```python
from build123d import *

# Parameters (mm, degrees)
EXTRUDE_1_DEPTH          = 40
SKETCH_2_R               = 3
CUT_EXTRUDE_1_DEPTH      = 14
SKETCH_3_R               = 4.25
CUT_EXTRUDE_2_DEPTH      = 33
CUT_EXTRUDE_2_DEPTH_BACK = 33
FILLET_1_R               = 15


with BuildPart() as part:
    # 草圖1 → 填料-伸長1 (new body)
    with BuildSketch(Plane.XY):
        with BuildLine():
            Line((-23, 35), (-32, 0))
            Line((-32, 0), (-25, 0))
            ThreePointArc((-25, 0), (0, 25), (25, 0))
            Line((25, 0), (32, 0))
            Line((32, 0), (23, 35))
            Line((23, 35), (23, 39))
            Line((23, 39), (-23, 39))
            Line((-23, 39), (-23, 35))
        make_face()
    extrude(amount=EXTRUDE_1_DEPTH)

    # 草圖2 → 除料-伸長1 (cut)
    with BuildSketch(Plane(origin=(0, 39, 0), x_dir=(1, 0, 0), z_dir=(0, 1, 0))):
        with Locations((-12, -20)):
            Circle(SKETCH_2_R)
        with Locations((12, -20)):
            Circle(SKETCH_2_R)
    extrude(amount=-CUT_EXTRUDE_1_DEPTH, mode=Mode.SUBTRACT)

    # 草圖3 → 除料-伸長2 (cut, two sides)
    with BuildSketch(Plane(origin=(0, 0, 0), x_dir=(0, 0, -1), z_dir=(1, 0, 0))) as cut_extrude_2_sk:
        with Locations((-20, 12)):
            Circle(SKETCH_3_R)
    extrude(amount=CUT_EXTRUDE_2_DEPTH, mode=Mode.SUBTRACT)
    extrude(cut_extrude_2_sk.sketch, amount=-CUT_EXTRUDE_2_DEPTH_BACK, mode=Mode.SUBTRACT)

    # 圓角1
    fillet_1_edges = [part.edges().sort_by_distance(p)[0] for p in [
        (-28.5, 0, 0),
        (-28.5, 0, 40),
        (28.5, 0, 40),
        (28.5, 0, 0),
    ]]
    fillet(fillet_1_edges, radius=FILLET_1_R)


solid = part.part
```
CAD build for the part. Positions are in the model's coordinates, mm. A direction names the side the tool comes from. Round coordinates to 2 decimals unless told otherwise and drop trailing zeros. Write each loop counter-clockwise with the first axis right and the second up, starting at its lowest first coordinate (ties: lowest second). Pieces come first, ordered by that corner, then holes. Notation, with made-up numbers: (-13, 5) -> (1, 5) arc R6 ccw to (1, 11) -> close; hole circle Ø4 at (3.5, 9). An arc over 180 degrees is marked (long way). Answer in a Markdown table with one row per item. Add a question column.
Item 1: Saw through at D-D, the plane x = 26.5. Write the cut outline in (y, z), then the cut area to 3 significant figures.
Item 2: Which spindle directions (+Z, -Z, +X, -X, +Y, -Y) get a long thin tool onto all of the face, cutting with end or side? Do faces 4 (the face through (0, 27, 0)), 5 (the face through (23, 37, 20)), 6 (the face through (-12, 25, 20)), 7 (the face through (-23, 37, 20)). Say none if no direction does.
Item 3: Drop flat-ended pins along their axis: pin 1 Ø8 at (x, y) = (22, 13) entering from +Z; pin 2 Ø2 at (y, z) = (31, 18.5) entering from -X; pin 3 Ø1.2 at (y, z) = (36, 20.5) entering from -X; pin 4 Ø8 at (y, z) = (14.5, 30.5) entering from -X. Give the stop position or say it passes through.
Item 4: Saw through at C-C, the plane y = 36.5. Write the cut outline in (x, z), then the cut area to 3 significant figures.
Item 5: Saw through at B-B, the plane z = 20. Write the cut outline in (x, y).
Item 6: Mould opens along Z. For faces 1 (the face through (11.35, 32.1, 22.93)), 2 (the face through (-27.25, 4.51, 4.28)), 3 (the face through (27.56, 17.26, 19.72)) say: pulls with the +Z half, pulls with the -Z half, needs draft (parallel to the pull), parting line crosses it, or undercut.
Item 7: Saw through at A-A, the plane y = 20. Write the cut outline in (x, z), then the cut area to 3 significant figures.
Item 8: Drill centre lines: line 1 (X direction, y = 35.75, z = 20); line 2 (Z direction, x = 12, y = 30.25); line 3 (Z direction, x = 10, y = 30). Where is each one in solid material? Low to high. Write a range as from..to.
Findings below:
| question | item | result |
|---|---|---|
| 1 | outline | (0, 15) arc R15 ccw to (15, 0) -> (21.39, 0) -> (21.39, 40) -> (15, 40) arc R15 ccw to (0, 25) -> close; hole circle Ø8.5 at (12, 20) |
| 1 | area | 702 mm^2 |
| 2 | face 4 | -Z, +X, -X, +Y, -Y |
| 2 | face 5 | +Z, -Z, +X, +Y |
| 2 | face 6 | +Y |
| 2 | face 7 | +Z, -Z, -X, +Y |
| 3 | pin 1 | stops at z = 40 |
| 3 | pin 2 | stops at x = -24.29 |
| 3 | pin 3 | stops at x = -23 |
| 3 | pin 4 | stops at x = -29.3 |
| 4 | outline | (-23, 0) -> (23, 0) -> (23, 40) -> (-23, 40) -> close; hole circle Ø6 at (-12, 20); hole circle Ø6 at (12, 20) |
| 4 | area | 1,780 mm^2 |
| 5 | outline | (-32, 0) -> (-25, 0) arc R25 cw to (-23.77, 7.75) -> (-30.01, 7.75) -> close; (-27.82, 16.25) -> (-19, 16.25) arc R25 cw to (19, 16.25) -> (27.82, 16.25) -> (23, 35) -> (23, 39) -> (15, 39) -> (15, 25) -> (9, 25) -> (9, 39) -> (-9, 39) -> (-9, 25) -> (-15, 25) -> (-15, 39) -> (-23, 39) -> (-23, 35) -> close; (23.77, 7.75) arc R25 cw to (25, 0) -> (32, 0) -> (30.01, 7.75) -> close |
| 6 | face 1 | undercut |
| 6 | face 2 | pulls with the -Z half |
| 6 | face 3 | needs draft |
| 7 | outline | (-26.86, 0) -> (-15, 0) -> (-15, 40) -> (-26.86, 40) -> close; (15, 0) -> (26.86, 0) -> (26.86, 40) -> (15, 40) -> close |
| 7 | area | 949 mm^2 |
| 8 | line 1 | x = -23..-15, -9..9, 15..23 |
| 8 | line 2 | z = 0..17, 23..40 |
| 8 | line 3 | z = 0..17.76, 22.24..40 |
